Geometry: final body of the model. Coordinates: model frame, mm. A direction names the side the tool comes from. Round coordinates to 2 decimals unless told otherwise and drop trailing zeros. Write each loop counter-clockwise with the first axis right and the second up, starting at its lowest first coordinate (ties: lowest second). Pieces come first, ordered by that corner, then holes. Notation, with made-up numbers: (-2, 16) -> (30, 16) arc R21 cw to (30, 34) -> close; hole circle Ø7 at (-35, 63.25). An arc over 180 degrees is marked (long way). One line per item, written item: value. Start each with the question number.
from build123d import *

# Parameters (mm, degrees)
BOSS_EXTRU_1_DEPTH      = 20
ESQUISSE3_R             = 1.5
ENL_V_MAT_EXTRU_3_DEPTH = 20
ESQUISSE4_R             = 1.5
ENL_V_MAT_EXTRU_4_DEPTH = 10
ESQUISSE5_R             = 1.5
ENL_V_MAT_EXTRU_5_DEPTH = 10
ESQUISSE6_R             = 1.4
BOSS_EXTRU_2_DEPTH      = 8.5


with BuildPart() as part:
    # Esquisse1 → Boss.-Extru.1 (new body)
    with BuildSketch(Plane(origin=(0, 0, 0), x_dir=(1, 0, 0), z_dir=(0, 1, 0))):
        with BuildLine():
            Line((-3, 84.398281038), (-3, 69.398281038))
            Line((-3, 69.398281038), (-7, 69.398281038))
            Line((-7, 69.398281038), (-7, 65.398281038))
            Line((-7, 65.398281038), (-3, 65.398281038))
            Line((-3, 65.398281038), (-3, 54.398281038))
            Line((-3, 54.398281038), (-18.71, 54.398281038))
            ThreePointArc((-18.71, 54.398281038), (-22.308577777, 49.499317693), (-26.183329952, 44.81574006))
            ThreePointArc((-26.183329952, 44.81574006), (-12.83252844, 48.159570073), (-5, 36.842476876))
            Line((-5, 36.842476876), (-5, -39.182739587))
            Line((-5, -39.182739587), (0, -39.182739587))
            Line((0, -39.182739587), (0, 84.398281038))
            Line((0, 84.398281038), (-3, 84.398281038))
        make_face()
    boss_extru_1 = extrude(amount=BOSS_EXTRU_1_DEPTH)

    # Symétrie1: Boss.-Extru.1 across plane
    add(boss_extru_1.mirror(Plane(origin=(0, 20, -84.398281038), x_dir=(0, 0, 1), z_dir=(-1, 0, 0))))

    # Esquisse3 → Enlèv. mat.-Extru.3 (cut)
    with BuildSketch(Plane.ZY.offset(3)):
        with Locations((-76.398281038, 10)):
            Circle(ESQUISSE3_R)
        with Locations((-60.398281038, 10)):
            Circle(ESQUISSE3_R)
    extrude(amount=-ENL_V_MAT_EXTRU_3_DEPTH, mode=Mode.SUBTRACT)

    # Esquisse4 → Enlèv. mat.-Extru.4 (cut)
    with BuildSketch(Plane.ZY.offset(5)):
        with Locations((29.291975875, 10.84)):
            Circle(ESQUISSE4_R)
    extrude(amount=-ENL_V_MAT_EXTRU_4_DEPTH, mode=Mode.SUBTRACT)

    # Esquisse5 → Enlèv. mat.-Extru.5 (cut)
    with BuildSketch(Plane.ZY.offset(5)):
        with Locations((17.841975875, 10.84)):
            Circle(ESQUISSE5_R)
    extrude(amount=-ENL_V_MAT_EXTRU_5_DEPTH, mode=Mode.SUBTRACT)

    # Esquisse6 → Boss.-Extru.2 (add)
    with BuildSketch(Plane(origin=(5, 0, 0), x_dir=(0, 0, -1), z_dir=(1, 0, 0))):
        with BuildLine():
            Line((5.308208853, 0), (-2.691791147, 0))
            Line((-2.691791147, 0), (-2.691791147, 35))
            ThreePointArc((-2.691791147, 35), (1.308208853, 39), (5.308208853, 35))
            Line((5.308208853, 35), (5.308208853, 0))
        make_face()
        with Locations((1.308208853, 35)):
            Circle(ESQUISSE6_R, mode=Mode.SUBTRACT)
    boss_extru_2 = extrude(amount=BOSS_EXTRU_2_DEPTH)

    # Symétrie2: Boss.-Extru.2 across plane
    add(boss_extru_2.mirror(Plane.ZY))


solid = part.part
(1) Set-up query: faces 1 (the face through (-11, 10, -54.398)), 2 (the face through (-5, 10, -69.398)), 3 (the face through (13.5, 20, -1)), 4 (the face through (5, 10, -65.398)). Return all of +Z, -Z, +X, -X, +Y, -Y with unobstructed straight access to the full face (end or side cutting, diameter ignored); none if empty.
(2) Pull-direction query (Z, two-part tool) for faces 5 (the face through (-5, 10, 21)), 6 (the face through (-0.042, 10.066, -77.897)), 7 (the face through (9.2, 39, -1.2)); classes: pulls with the +Z half, pulls with the -Z half, needs draft (parallel to the pull), parting line crosses it, or undercut.
(3) Section query A-A (y = 25). Output: boundary loops of the cut face in (x, z).
(4) Line query: probe 1 along X at (y, z) = (6, 7); probe 2 along Z at (x, y) = (-10.5, 19.5); probe 3 along Y at (x, z) = (4, -68). Output: solid intervals per line, ascending.
(5) Pin query (flat end, axial travel): pin 1 (10 mm diameter, centred on y = 8, z = -17.5, fed in from -X); pin 2 (8 mm diameter, centred on x = -2, z = 1, fed in from +Y); pin 3 (4.5 mm diameter, centred on y = 10.5, z = -67.5, fed in from -X); pin 4 (9 mm diameter, centred on y = 10, z = -3, fed in from +X). Return the tip coordinate at first contact, or that it passes through.
(6) Section query C-C (z = -42.5). Output: boundary loops of the cut face in (x, y).
Results list:
1. face 1: -X, +Y, -Y
1. face 2: -Z, -X, +Y, -Y
1. face 3: +Z, +X, +Y, -Y
1. face 4: +X, +Y, -Y
2. face 5: needs draft
2. face 6: undercut
2. face 7: parting line crosses it
3. outline: (-13.5, -5.31) -> (-5, -5.31) -> (-5, 2.69) -> (-13.5, 2.69) -> close; (5, -5.31) -> (13.5, -5.31) -> (13.5, 2.69) -> (5, 2.69) -> close
4. probe 1: x = -5 to 5
4. probe 2: z = -54.4 to -46.98, -5.31 to 2.69
4. probe 3: y = 0 to 20
5. pin 1: stops at x = -5
5. pin 2: stops at y = 39
5. pin 3: stops at x = -7
5. pin 4: stops at x = 13.5
6. outline: (-6.41, 0) -> (6.41, 0) -> (6.41, 20) -> (-6.41, 20) -> close
